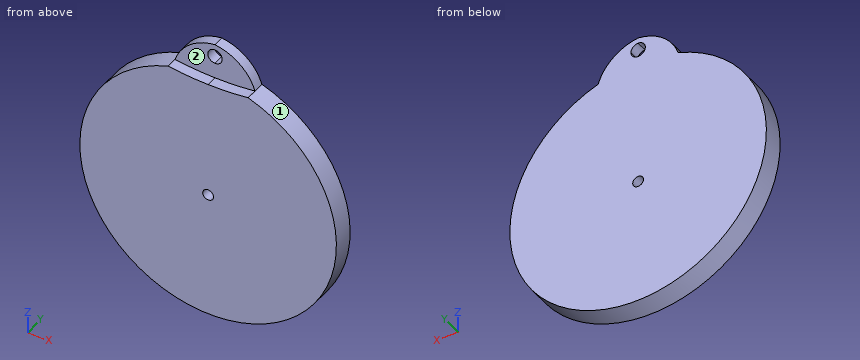
```python
from build123d import *

# Parameters (mm, degrees)
F1_DEPTH = 3
F2_DEPTH = 6


# Not quite as in the source:
# - the program builds the solid bodies; features that only make, move or delete a surface that nothing else refers to are left out


with BuildPart() as f1:
    # F0 (on Front) → F1 (new body)
    with BuildSketch(Plane.XZ):
        with BuildLine():
            ThreePointArc((-36.2547188994, 42.8754752639), (-41.8166946482, 43.071513271), (-47.3510663807, 43.6586543583))
            ThreePointArc((-47.3510663807, 43.6586543583), (-36.2547188994, -25.6966625147), (-25.1583714182, 43.6586543583))
            ThreePointArc((-25.1583714182, 43.6586543583), (-30.6927431507, 43.071513271), (-36.2547188994, 42.8754752639))
        make_face()
        with BuildLine():
            ThreePointArc((-34.7547188994, 9.8686634646), (-37.3153790712, 8.8080032929), (-36.2547188994, 11.3686634646))
            ThreePointArc((-36.2547188994, 11.3686634646), (-35.1940587277, 10.9293236364), (-34.7547188994, 9.8686634646))
        make_face(mode=Mode.SUBTRACT)
        with BuildLine():
            ThreePointArc((-36.2547188994, 52.7826075633), (-43.1513282612, 49.8605681538), (-47.3510663807, 43.6586543583))
            ThreePointArc((-47.3510663807, 43.6586543583), (-41.8166946482, 43.071513271), (-36.2547188994, 42.8754752639))
            Line((-36.2547188994, 42.8754752639), (-36.2547188994, 47.2246634646))
            ThreePointArc((-36.2547188994, 47.2246634646), (-38.2547188994, 49.2246634646), (-36.2547188994, 51.2246634646))
            Line((-36.2547188994, 51.2246634646), (-36.2547188994, 52.7826075633))
        make_face()
        with BuildLine():
            ThreePointArc((-36.2547188994, 42.8754752639), (-30.6927431507, 43.071513271), (-25.1583714182, 43.6586543583))
            ThreePointArc((-25.1583714182, 43.6586543583), (-29.3581095377, 49.8605681538), (-36.2547188994, 52.7826075633))
            Line((-36.2547188994, 52.7826075633), (-36.2547188994, 51.2246634646))
            ThreePointArc((-36.2547188994, 51.2246634646), (-34.8405053371, 50.638877027), (-34.2547188994, 49.2246634646))
            ThreePointArc((-34.2547188994, 49.2246634646), (-34.8405053371, 47.8104499023), (-36.2547188994, 47.2246634646))
            Line((-36.2547188994, 47.2246634646), (-36.2547188994, 42.8754752639))
        make_face()
    extrude(amount=F1_DEPTH)

    # F0 (on Front) → F2 (join)
    with BuildSketch(Plane.XZ):
        with BuildLine():
            ThreePointArc((-36.2547188994, 42.8754752639), (-41.8166946482, 43.071513271), (-47.3510663807, 43.6586543583))
            ThreePointArc((-47.3510663807, 43.6586543583), (-36.2547188994, -25.6966625147), (-25.1583714182, 43.6586543583))
            ThreePointArc((-25.1583714182, 43.6586543583), (-30.6927431507, 43.071513271), (-36.2547188994, 42.8754752639))
        make_face()
        with BuildLine():
            ThreePointArc((-34.7547188994, 9.8686634646), (-37.3153790712, 8.8080032929), (-36.2547188994, 11.3686634646))
            ThreePointArc((-36.2547188994, 11.3686634646), (-35.1940587277, 10.9293236364), (-34.7547188994, 9.8686634646))
        make_face(mode=Mode.SUBTRACT)
    extrude(amount=F2_DEPTH)


solid = f1.part
```
CAD build for the part. Positions are in the model's coordinates, mm. Face numbers are marked on the shaded views. A direction names the side the tool comes from. Round coordinates to 2 decimals unless told otherwise and drop trailing zeros. Loops run counter-clockwise (first coordinate to the right, second up) from the corner with the lowest first, then second, coordinate; pieces in that order, holes last. Notation, with made-up numbers: (58, -20.75) - (90, -20.75) arc R26 cw to (90, -0.75) - close; hole circle Ø3 at (70, 27). An arc over 180 degrees is marked (long way). Return JSON: item names as keys, results as strings. Group by question number.
Q1. Band-saw the part on A-A on y = -1.65. Give the cut face in (x, z).
Q2. Band-saw the part on B-B on z = -16. Give the cut face in (x, y).
Q3. Flat gauge pins, fed straight in: pin 1 Ø1 at (x, y) = (-30, -2.5) entering from +Z; pin 2 Ø2 at (y, z) = (-2, 28.5) entering from +X; pin 3 Ø3 at (x, z) = (-35, 46) entering from -Y. Where does each tip first touch, or does it go through?
Q4. Tool access for the marked faces 1 and 2: list every direction of +Z, -Z, +X, -X, +Y, -Y with a clear straight run to the whole face (end or side of a thin tool).
Q5. Drill centre lines: line 1 along X through (y, z) = (-1.8, 10); line 2 along X through (y, z) = (-0.95, 9); line 3 along Z through (x, y) = (-31, -4.25). Where is each one in solid material? Low to high. Write a range as [from, to].
Q6. Band-saw the part on C-C on x = -5.5. Give the cut face in (y, z).
Solutions:
{
 "1": {"outline": "(-47.35, 43.66) arc R35.57 ccw (long way) to (-25.16, 43.66) arc R13.21 ccw to (-36.25, 52.78) arc R13.21 ccw to start; hole circle Ø4 at (-36.25, 49.22); hole circle Ø3 at (-36.25, 9.87)"},
 "2": {"outline": "(-60.66, -6) - (-11.85, -6) - (-11.85, 0) - (-60.66, 0) - close"},
 "3": {"pin 1": "stops at z = 50.7", "pin 2": "stops at x = -5.37", "pin 3": "stops at y = -3"},
 "4": {"face 1": "+Y, -Y", "face 2": "+Z, -Y"},
 "5": {"line 1": "x = [-71.82, -37.75], [-34.76, -0.69]", "line 2": "x = [-71.81, -37.48], [-35.03, -0.7]", "line 3": "z = [-25.31, 43.05]"},
 "6": {"outline": "(-6, -7.99) - (0, -7.99) - (0, 27.73) - (-6, 27.73) - close"}
}
